Work out the finished part from the listing and answer in its coordinate system (mm). Give positions to 0.01 mm unless a question says otherwise; leave off trailing zeros. Write each loop counter-clockwise with the first axis right and the second up, starting at its lowest first coordinate (ties: lowest second). Pieces come first, ordered by that corner, then holes. Notation, with made-up numbers: (59, 74.25) - (108, 74.25) arc R10 cw to (108, 92.25) - close; hole circle Ø3 at (82.25, 9.5). An arc over 180 degrees is marked (long way). Write each question's results on one line, items separated by ' | '. Start each with the question number.
from build123d import *

# Parameters (mm, degrees)
SKETCH1_W           = 4.953
SKETCH1_H           = 58.42
SKETCH1_W_2         = 1.27
SKETCH1_H_2         = 1.27
BOSS_EXTRUDE1_DEPTH = 7.62


with BuildPart() as part:
    # Sketch1 → Boss-Extrude1 (new body)
    with BuildSketch(Plane(origin=(0, 0, 0), x_dir=(1, 0, 0), z_dir=(0, 1, 0))):
        with Locations((2.4765, 29.21)):
            Rectangle(SKETCH1_W, SKETCH1_H)
        with Locations((3.691399704, 57.15)):
            Rectangle(SKETCH1_W_2, SKETCH1_H_2, mode=Mode.SUBTRACT)
        with Locations((1.151399704, 57.15)):
            Rectangle(SKETCH1_W_2, SKETCH1_H_2, mode=Mode.SUBTRACT)
        with Locations((3.691399704, 54.61)):
            Rectangle(SKETCH1_W_2, SKETCH1_H_2, mode=Mode.SUBTRACT)
        with Locations((1.151399704, 54.648853122)):
            Rectangle(SKETCH1_W_2, SKETCH1_H_2, mode=Mode.SUBTRACT)
        with Locations((3.691399704, 52.07)):
            Rectangle(SKETCH1_W_2, SKETCH1_H_2, mode=Mode.SUBTRACT)
        with Locations((1.151399704, 52.07)):
            Rectangle(SKETCH1_W_2, SKETCH1_H_2, mode=Mode.SUBTRACT)
        with Locations((3.691399704, 49.53)):
            Rectangle(SKETCH1_W_2, SKETCH1_H_2, mode=Mode.SUBTRACT)
        with Locations((1.151399704, 49.568853122)):
            Rectangle(SKETCH1_W_2, SKETCH1_H_2, mode=Mode.SUBTRACT)
        with Locations((3.691399704, 46.99)):
            Rectangle(SKETCH1_W_2, SKETCH1_H_2, mode=Mode.SUBTRACT)
        with Locations((1.151399704, 46.99)):
            Rectangle(SKETCH1_W_2, SKETCH1_H_2, mode=Mode.SUBTRACT)
        with Locations((3.691399704, 44.45)):
            Rectangle(SKETCH1_W_2, SKETCH1_H_2, mode=Mode.SUBTRACT)
        with Locations((1.151399704, 44.488853122)):
            Rectangle(SKETCH1_W_2, SKETCH1_H_2, mode=Mode.SUBTRACT)
        with Locations((3.691399704, 41.91)):
            Rectangle(SKETCH1_W_2, SKETCH1_H_2, mode=Mode.SUBTRACT)
        with Locations((1.151399704, 41.91)):
            Rectangle(SKETCH1_W_2, SKETCH1_H_2, mode=Mode.SUBTRACT)
        with Locations((3.691399704, 39.37)):
            Rectangle(SKETCH1_W_2, SKETCH1_H_2, mode=Mode.SUBTRACT)
        with Locations((1.151399704, 39.408853122)):
            Rectangle(SKETCH1_W_2, SKETCH1_H_2, mode=Mode.SUBTRACT)
        with Locations((3.691399704, 36.83)):
            Rectangle(SKETCH1_W_2, SKETCH1_H_2, mode=Mode.SUBTRACT)
        with Locations((1.151399704, 36.83)):
            Rectangle(SKETCH1_W_2, SKETCH1_H_2, mode=Mode.SUBTRACT)
        with Locations((3.691399704, 34.29)):
            Rectangle(SKETCH1_W_2, SKETCH1_H_2, mode=Mode.SUBTRACT)
        with Locations((1.151399704, 34.328853122)):
            Rectangle(SKETCH1_W_2, SKETCH1_H_2, mode=Mode.SUBTRACT)
        with Locations((3.691399704, 31.75)):
            Rectangle(SKETCH1_W_2, SKETCH1_H_2, mode=Mode.SUBTRACT)
        with Locations((1.151399704, 31.75)):
            Rectangle(SKETCH1_W_2, SKETCH1_H_2, mode=Mode.SUBTRACT)
        with Locations((3.691399704, 29.21)):
            Rectangle(SKETCH1_W_2, SKETCH1_H_2, mode=Mode.SUBTRACT)
        with Locations((1.151399704, 29.248853122)):
            Rectangle(SKETCH1_W_2, SKETCH1_H_2, mode=Mode.SUBTRACT)
        with Locations((3.691399704, 26.67)):
            Rectangle(SKETCH1_W_2, SKETCH1_H_2, mode=Mode.SUBTRACT)
        with Locations((1.151399704, 26.67)):
            Rectangle(SKETCH1_W_2, SKETCH1_H_2, mode=Mode.SUBTRACT)
        with Locations((3.691399704, 24.13)):
            Rectangle(SKETCH1_W_2, SKETCH1_H_2, mode=Mode.SUBTRACT)
        with Locations((1.151399704, 24.168853122)):
            Rectangle(SKETCH1_W_2, SKETCH1_H_2, mode=Mode.SUBTRACT)
        with Locations((3.691399704, 21.59)):
            Rectangle(SKETCH1_W_2, SKETCH1_H_2, mode=Mode.SUBTRACT)
        with Locations((1.151399704, 21.59)):
            Rectangle(SKETCH1_W_2, SKETCH1_H_2, mode=Mode.SUBTRACT)
        with Locations((3.691399704, 19.05)):
            Rectangle(SKETCH1_W_2, SKETCH1_H_2, mode=Mode.SUBTRACT)
        with Locations((1.151399704, 19.088853122)):
            Rectangle(SKETCH1_W_2, SKETCH1_H_2, mode=Mode.SUBTRACT)
        with Locations((3.691399704, 16.51)):
            Rectangle(SKETCH1_W_2, SKETCH1_H_2, mode=Mode.SUBTRACT)
        with Locations((1.151399704, 16.51)):
            Rectangle(SKETCH1_W_2, SKETCH1_H_2, mode=Mode.SUBTRACT)
        with Locations((3.691399704, 13.97)):
            Rectangle(SKETCH1_W_2, SKETCH1_H_2, mode=Mode.SUBTRACT)
        with Locations((1.151399704, 14.008853122)):
            Rectangle(SKETCH1_W_2, SKETCH1_H_2, mode=Mode.SUBTRACT)
        with Locations((3.691399704, 11.43)):
            Rectangle(SKETCH1_W_2, SKETCH1_H_2, mode=Mode.SUBTRACT)
        with Locations((1.151399704, 11.43)):
            Rectangle(SKETCH1_W_2, SKETCH1_H_2, mode=Mode.SUBTRACT)
        with Locations((3.691399704, 8.89)):
            Rectangle(SKETCH1_W_2, SKETCH1_H_2, mode=Mode.SUBTRACT)
        with Locations((1.151399704, 8.928853122)):
            Rectangle(SKETCH1_W_2, SKETCH1_H_2, mode=Mode.SUBTRACT)
        with Locations((3.691399704, 6.35)):
            Rectangle(SKETCH1_W_2, SKETCH1_H_2, mode=Mode.SUBTRACT)
        with Locations((1.151399704, 6.35)):
            Rectangle(SKETCH1_W_2, SKETCH1_H_2, mode=Mode.SUBTRACT)
        with Locations((3.691399704, 3.81)):
            Rectangle(SKETCH1_W_2, SKETCH1_H_2, mode=Mode.SUBTRACT)
        with Locations((1.151399704, 3.848853122)):
            Rectangle(SKETCH1_W_2, SKETCH1_H_2, mode=Mode.SUBTRACT)
        with Locations((3.691399704, 1.27)):
            Rectangle(SKETCH1_W_2, SKETCH1_H_2, mode=Mode.SUBTRACT)
        with Locations((1.151399704, 1.308853122)):
            Rectangle(SKETCH1_W_2, SKETCH1_H_2, mode=Mode.SUBTRACT)
    extrude(amount=BOSS_EXTRUDE1_DEPTH)


solid = part.part
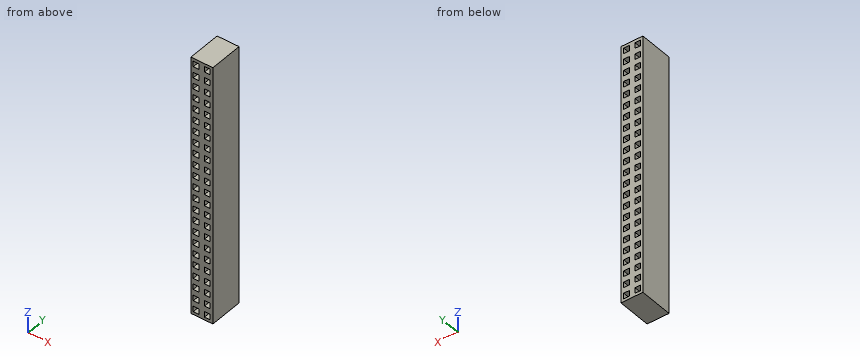
Q1. Consider L1, parallel to X at y = 0.5, z = -19.5. Determine where the line is inside the solid, lowest interval first.
Q2. A cutting plane is placed at A-A, the plane z = -42. Write down the section's boundary in (x, y), and give its area (3 significant figures).
Q3. A cutting plane is placed at B-B, the plane x = 1.1. Give the number of separate pieces and of enclosed holes in the cut face, and give its area (3 significant figures).
Result:
1) L1: x = 0 to 0.52, 1.79 to 3.06, 4.33 to 4.95
2) outline: (0, 0) - (0.52, 0) - (0.52, 7.62) - (0, 7.62) - close; (1.79, 0) - (3.06, 0) - (3.06, 7.62) - (1.79, 7.62) - close; (4.33, 0) - (4.95, 0) - (4.95, 7.62) - (4.33, 7.62) - close | area: 18.4 mm2
3) separate pieces: 24 | enclosed holes: 0 | area: 223 mm2
